Design review of the part built by this model. Coordinates are the model's own, in mm. A direction names the side the tool comes from. Coordinates: 2 decimals unless noted, no trailing zeros. Loops run counter-clockwise (first coordinate to the right, second up) from the corner with the lowest first, then second, coordinate; pieces in that order, holes last. Notation, with made-up numbers: M 87.25,76.5 L 140.25,76.5 A24 ccw 140.25,97.5 Z; hole C 1.5,27 d11. An arc over 180 degrees is marked long. One line per item, written item: value.
```python
from build123d import *

# Parameters (mm, degrees)
CROQUIS1_R              = 19.85
SALIENTE_EXTRUIR1_DEPTH = 6
CROQUIS2_R              = 30
SALIENTE_EXTRUIR3_DEPTH = 2
CROQUIS3_W              = 2.5
CROQUIS3_H              = 34
SALIENTE_EXTRUIR4_DEPTH = 20
CROQUIS4_W              = 2.5
CROQUIS4_H              = 10
SALIENTE_EXTRUIR5_DEPTH = 5
CROQUIS5_W              = 23
CROQUIS5_H              = 34
SALIENTE_EXTRUIR6_DEPTH = 5
CORTAR_EXTRUIR1_REACH   = 64.65
CROQUIS6_R              = 1
CORTAR_EXTRUIR3_REACH   = 55.749
CROQUIS8_R              = 1
CROQUIS10_R             = 3
CROQUIS10_R_2           = 1.25
SALIENTE_EXTRUIR8_DEPTH = 28
REDONDEO1_R             = 3
CROQUIS11_R             = 4.5
CORTAR_EXTRUIR5_DEPTH   = 10
REDONDEO2_R             = 1
CROQUIS12_R             = 2.3
CORTAR_EXTRUIR6_DEPTH   = 11


with BuildPart() as part:
    # Croquis1 → Saliente-Extruir1 (new body)
    with BuildSketch(Plane.XY):
        Circle(CROQUIS1_R)
    extrude(amount=SALIENTE_EXTRUIR1_DEPTH)

    # Croquis2 → Saliente-Extruir3 (add)
    with BuildSketch(Plane.XY.offset(6)):
        Circle(CROQUIS2_R)
    extrude(amount=SALIENTE_EXTRUIR3_DEPTH)

    # Croquis3 → Saliente-Extruir4 (add)
    with BuildSketch(Plane.XY.offset(8)):
        with Locations((-12.75, 0)):
            Rectangle(CROQUIS3_W, CROQUIS3_H)
    extrude(amount=SALIENTE_EXTRUIR4_DEPTH)

    # Croquis4 → Saliente-Extruir5 (add)
    with BuildSketch(Plane.XY.offset(28)):
        with Locations((-12.75, 12)):
            Rectangle(CROQUIS4_W, CROQUIS4_H)
        with Locations((-12.75, -12)):
            Rectangle(CROQUIS4_W, CROQUIS4_H)
    extrude(amount=SALIENTE_EXTRUIR5_DEPTH)

    # Croquis5 → Saliente-Extruir6 (add)
    with BuildSketch(Plane.XY.offset(8)):
        Rectangle(CROQUIS5_W, CROQUIS5_H)
    extrude(amount=SALIENTE_EXTRUIR6_DEPTH)

    # Croquis6 → Cortar-Extruir1 (cut, up to next)
    with BuildSketch(Plane.ZY.offset(14), mode=Mode.PRIVATE) as cortar_extruir1_sk1:
        with Locations((15, -15)):
            Circle(CROQUIS6_R)
    cortar_extruir1_tool1 = extrude(cortar_extruir1_sk1.sketch, amount=-CORTAR_EXTRUIR1_REACH, mode=Mode.PRIVATE) & part.part
    # Croquis6 → Cortar-Extruir1 (cut, up to next)
    with BuildSketch(Plane.ZY.offset(14), mode=Mode.PRIVATE) as cortar_extruir1_sk2:
        with Locations((31, -15)):
            Circle(CROQUIS6_R)
    cortar_extruir1_tool2 = extrude(cortar_extruir1_sk2.sketch, amount=-CORTAR_EXTRUIR1_REACH, mode=Mode.PRIVATE) & part.part
    # Croquis6 → Cortar-Extruir1 (cut, up to next)
    with BuildSketch(Plane.ZY.offset(14), mode=Mode.PRIVATE) as cortar_extruir1_sk3:
        with Locations((15, 15)):
            Circle(CROQUIS6_R)
    cortar_extruir1_tool3 = extrude(cortar_extruir1_sk3.sketch, amount=-CORTAR_EXTRUIR1_REACH, mode=Mode.PRIVATE) & part.part
    # Croquis6 → Cortar-Extruir1 (cut, up to next)
    with BuildSketch(Plane.ZY.offset(14), mode=Mode.PRIVATE) as cortar_extruir1_sk4:
        with Locations((31, 15)):
            Circle(CROQUIS6_R)
    cortar_extruir1_tool4 = extrude(cortar_extruir1_sk4.sketch, amount=-CORTAR_EXTRUIR1_REACH, mode=Mode.PRIVATE) & part.part
    add(cortar_extruir1_tool1.solids().sort_by_distance((-14, -15, 15))[0], mode=Mode.SUBTRACT)
    add(cortar_extruir1_tool2.solids().sort_by_distance((-14, -15, 31))[0], mode=Mode.SUBTRACT)
    add(cortar_extruir1_tool3.solids().sort_by_distance((-14, 15, 15))[0], mode=Mode.SUBTRACT)
    add(cortar_extruir1_tool4.solids().sort_by_distance((-14, 15, 31))[0], mode=Mode.SUBTRACT)

    # Croquis8 → Cortar-Extruir3 (cut, up to next)
    with BuildSketch(Plane(origin=(0, 0, 0), x_dir=(-1, 0, 0), z_dir=(0, 0, -1)), mode=Mode.PRIVATE) as cortar_extruir3_sk1:
        with Locations((0.001043545, -5.999999909)):
            Circle(CROQUIS8_R)
    cortar_extruir3_tool1 = extrude(cortar_extruir3_sk1.sketch, amount=-CORTAR_EXTRUIR3_REACH, mode=Mode.PRIVATE) & part.part
    # Croquis8 → Cortar-Extruir3 (cut, up to next)
    with BuildSketch(Plane(origin=(0, 0, 0), x_dir=(-1, 0, 0), z_dir=(0, 0, -1)), mode=Mode.PRIVATE) as cortar_extruir3_sk2:
        with Locations((-5.999999909, -0.001043545)):
            Circle(CROQUIS8_R)
    cortar_extruir3_tool2 = extrude(cortar_extruir3_sk2.sketch, amount=-CORTAR_EXTRUIR3_REACH, mode=Mode.PRIVATE) & part.part
    # Croquis8 → Cortar-Extruir3 (cut, up to next)
    with BuildSketch(Plane(origin=(0, 0, 0), x_dir=(-1, 0, 0), z_dir=(0, 0, -1)), mode=Mode.PRIVATE) as cortar_extruir3_sk3:
        with Locations((-0.001043545, 5.999999909)):
            Circle(CROQUIS8_R)
    cortar_extruir3_tool3 = extrude(cortar_extruir3_sk3.sketch, amount=-CORTAR_EXTRUIR3_REACH, mode=Mode.PRIVATE) & part.part
    # Croquis8 → Cortar-Extruir3 (cut, up to next)
    with BuildSketch(Plane(origin=(0, 0, 0), x_dir=(-1, 0, 0), z_dir=(0, 0, -1)), mode=Mode.PRIVATE) as cortar_extruir3_sk4:
        with Locations((5.999999909, 0.001043545)):
            Circle(CROQUIS8_R)
    cortar_extruir3_tool4 = extrude(cortar_extruir3_sk4.sketch, amount=-CORTAR_EXTRUIR3_REACH, mode=Mode.PRIVATE) & part.part
    add(cortar_extruir3_tool1.solids().sort_by_distance((-0.001044, -6, 0))[0], mode=Mode.SUBTRACT)
    add(cortar_extruir3_tool2.solids().sort_by_distance((6, -0.001044, 0))[0], mode=Mode.SUBTRACT)
    add(cortar_extruir3_tool3.solids().sort_by_distance((0.001044, 6, 0))[0], mode=Mode.SUBTRACT)
    add(cortar_extruir3_tool4.solids().sort_by_distance((-6, 0.001044, 0))[0], mode=Mode.SUBTRACT)

    # Croquis10 → Saliente-Extruir8 (add)
    # profile 1 of 3: a face of its own
    with BuildSketch(Plane.XY.offset(8)):
        with Locations((0, 23.5)):
            Circle(CROQUIS10_R)
        with Locations((0, 23.5)):
            Circle(CROQUIS10_R_2, mode=Mode.SUBTRACT)
    # profile 2 of 3: a face of its own
    with BuildSketch(Plane.XY.offset(8)):
        with Locations((0, -23.5)):
            Circle(CROQUIS10_R)
        with Locations((0, -23.5)):
            Circle(CROQUIS10_R_2, mode=Mode.SUBTRACT)
    # profile 3 of 3: a face of its own
    with BuildSketch(Plane.XY.offset(8)):
        with Locations((-22, 0)):
            Circle(CROQUIS10_R)
        with Locations((-22, 0)):
            Circle(CROQUIS10_R_2, mode=Mode.SUBTRACT)
    extrude(amount=SALIENTE_EXTRUIR8_DEPTH)

    # Redondeo1
    redondeo1_edges = [part.edges().sort_by_distance(p)[0] for p in [
        (-3, 23.5, 8),
        (-3, -23.5, 8),
        (-25, 0, 8),
    ]]
    fillet(redondeo1_edges, radius=REDONDEO1_R)

    # Croquis11 → Cortar-Extruir5 (cut)
    with BuildSketch(Plane(origin=(0, 0, 0), x_dir=(-1, 0, 0), z_dir=(0, 0, -1))):
        with Locations((13.999999486, 0.002434939)):
            Circle(CROQUIS11_R)
    extrude(amount=-CORTAR_EXTRUIR5_DEPTH, mode=Mode.SUBTRACT)

    # Redondeo2
    redondeo2_edges = [part.edges().sort_by_distance(p)[0] for p in [
        (-14, 0.002434939, 10),
        (-14, -4.497565061, 9),
        (-14, 4.502434939, 9),
    ]]
    fillet(redondeo2_edges, radius=REDONDEO2_R)

    # Croquis12 → Cortar-Extruir6 (cut)
    with BuildSketch(Plane.XY.offset(13)):
        with Locations((5.999999909, -0.001043545)):
            Circle(CROQUIS12_R)
        with Locations((-0.001043545, -5.999999909)):
            Circle(CROQUIS12_R)
        with Locations((-5.999999909, 0.001043545)):
            Circle(CROQUIS12_R)
        with Locations((0.001043545, 5.999999909)):
            Circle(CROQUIS12_R)
    extrude(amount=-CORTAR_EXTRUIR6_DEPTH, mode=Mode.SUBTRACT)


solid = part.part
```
(1) Mouldability with a two-part tool opening along X and no side actions: class faces 1 (the flat face through (11.5, 0, 10)), 2 (the cylindrical face through (-25, 0, 23)), 3 (the flat face through (-13, 0, 28)) as released by +X, released by -X, zero draft, split by the parting line, or undercut.
Reply:
face 1: released by +X
face 2: undercut
face 3: zero draft
(2) We need section B-B on z = 15. State how many separate pieces and enclosed holes the cut face has, then the cut area to 3 significant figures.
Reply:
separate pieces: 6
enclosed holes: 3
area: 145 mm2
(3) We need section A-A on z = 27. State the section outline as (x, y) points, then the cut area to 3 significant figures.
Reply:
outline: C -22,0 d6; M -14,-17 L -11.5,-17 L -11.5,17 L -14,17 Z; C 0,-23.5 d6; C 0,23.5 d6; hole C -22,0 d2.5; hole C 0,-23.5 d2.5; hole C 0,23.5 d2.5
area: 155 mm2
(4) We need section D-D on y = -15. State the section outline as (x, z) points, then the cut area to 3 significant figures.
Reply:
outline: M -25.98,6 L -13,6 L -13,0 L 13,0 L 13,6 L 25.98,6 L 25.98,8 L 11.5,8 L 11.5,13 L -11.5,13 L -11.5,14 L -14,14 L -14,8 L -25.98,8 Z; M -14,16 L -11.5,16 L -11.5,30 L -14,30 Z; M -14,32 L -11.5,32 L -11.5,33 L -14,33 Z
area: 427 mm2
(5) Insertion check: pin 1 (5 mm diameter, centred on x = -0.5, y = -6, fed in from +Z); pin 2 (0.8 mm diameter, centred on x = -22, y = 0.5, fed in from +Z); pin 3 (5 mm diameter, centred on x = -2.5, z = 31, fed in from -Y). Each pin has a flat end and moves straight along its axis. Give the tip position at first contact, or say it passes through.
Reply:
pin 1: stops at z = 13
pin 2: stops at z = 8
pin 3: stops at y = -26.5
(6) Tool access review of faces 4 (the flat face through (-13, -7, 30)), 5 (the cylindrical face through (-10.4, -2.7, 4.9)), 6 (the flat face through (-1, 5, 2)): name each direction out of +Z, -Z, +X, -X, +Y, -Y from which nothing blocks a thin tool from reaching the whole face with its end or side.
Reply:
face 4: +Z, +X, -X
face 5: -Z
face 6: +Z
(7) To check wall thickness, follow line 1 along Y through (x, z) = (0, 30.5); line 2 along X through (y, z) = (1, 25.5); line 3 along Z through (x, y) = (-18, 2.5). State the ranges of each line that lie inside material, in increasing order. Write a range as [from, to].
Reply:
line 1: y = [-26.5, -24.75], [-22.25, -20.5], [20.5, 22.25], [24.75, 26.5]
line 2: x = [-24.83, -22.75], [-21.25, -19.17], [-14, -11.5]
line 3: z = [0, 8.29]
